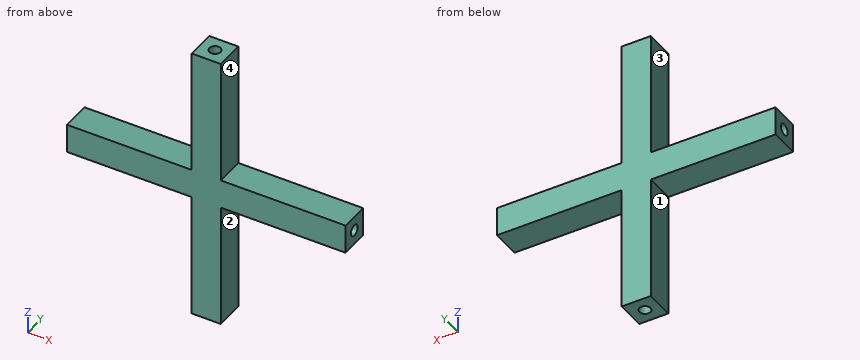
from build123d import *

# Parameters (mm, degrees)
BOSS_EXTRUDE1_DEPTH = 1.75
CUT_EXTRUDE4_START  = -1.75
SKETCH2_R           = 0.675
CUT_EXTRUDE4_DEPTH  = 16
CUT_EXTRUDE5_START  = 1.75
SKETCH2_2_R         = 0.675
CUT_EXTRUDE5_DEPTH  = 16
CUT_EXTRUDE6_START  = 1.75
SKETCH3_R           = 0.675
CUT_EXTRUDE6_DEPTH  = 16
CUT_EXTRUDE7_START  = -1.75
SKETCH3_2_R         = 0.675
CUT_EXTRUDE7_DEPTH  = 16


with BuildPart() as part:
    # Sketch1 → Boss-Extrude1 (new body, symmetric)
    with BuildSketch(Plane(origin=(0, 0, 0), x_dir=(1, 0, 0), z_dir=(0, 1, 0))):
        Polygon((1.75, -1.75), (1.75, -16.75), (-1.75, -16.75), (-1.75, -1.75), (-16.75, -1.75), (-16.75, 1.75), (-1.75, 1.75), (-1.75, 16.75), (1.75, 16.75), (1.75, 1.75), (16.75, 1.75), (16.75, -1.75), align=None)
    extrude(amount=BOSS_EXTRUDE1_DEPTH, both=True)

    # Sketch2 → Cut-Extrude4 (cut, through all)
    with BuildSketch(Plane.XY.offset(CUT_EXTRUDE4_START)):
        Circle(SKETCH2_R)
    extrude(amount=-CUT_EXTRUDE4_DEPTH, mode=Mode.SUBTRACT)

    # Sketch2<2> → Cut-Extrude5 (cut, through all)
    with BuildSketch(Plane.XY.offset(CUT_EXTRUDE5_START)):
        Circle(SKETCH2_2_R)
    extrude(amount=CUT_EXTRUDE5_DEPTH, mode=Mode.SUBTRACT)

    # Sketch3 → Cut-Extrude6 (cut, through all)
    with BuildSketch(Plane.ZY.offset(CUT_EXTRUDE6_START)):
        Circle(SKETCH3_R)
    extrude(amount=CUT_EXTRUDE6_DEPTH, mode=Mode.SUBTRACT)

    # Sketch3<2> → Cut-Extrude7 (cut, through all)
    with BuildSketch(Plane.ZY.offset(CUT_EXTRUDE7_START)):
        Circle(SKETCH3_2_R)
    extrude(amount=-CUT_EXTRUDE7_DEPTH, mode=Mode.SUBTRACT)


solid = part.part
Design review of the part built by this model. Coordinates are the model's own, in mm. Face numbers are marked on the shaded views. A direction names the side the tool comes from. Give positions to 0.01 mm unless a question says otherwise; leave off trailing zeros. Loops run counter-clockwise (first coordinate to the right, second up) from the corner with the lowest first, then second, coordinate; pieces in that order, holes last. Notation, with made-up numbers: M -38,-10 L -18,-10 A23 ccw -18,10 Z; hole C -16.75,33 d11. An arc over 180 degrees is marked long. Answer as a JSON object with one key per item and string values.
Item 1: We need section C-C (x = 0). State the section outline as (y, z) points (3 decimals).
Output values:
{"outline": "M -1.75,-16.75 L -0.675,-16.75 L -0.675,-1.75 L 0.675,-1.75 L 0.675,-16.75 L 1.75,-16.75 L 1.75,16.75 L 0.675,16.75 L 0.675,1.75 L -0.675,1.75 L -0.675,16.75 L -1.75,16.75 Z"}
Item 2: For P1, Ø0.8, axis at x = 0, y = 0, coming from the +Z side; P2, Ø1.1, axis at y = 0, z = 0, coming from the +X side; P3, Ø5, axis at x = -3, z = -7.5, coming from the -Y side; P4, Ø1.5, axis at y = 0.5, z = 9.5, coming from the -X side, all flat-tipped, find the tip position at first contact; note any pin that passes through.
Output values:
{"P1": "stops at z = 1.75", "P2": "stops at x = 1.75", "P3": "stops at y = -1.75", "P4": "stops at x = -1.75"}
Item 3: We need section D-D (z = 0). State the section outline as (x, y) points (3 decimals), and give its area (4 significant figures).
Output values:
{"outline": "M -16.75,-1.75 L 16.75,-1.75 L 16.75,-0.675 L 1.75,-0.675 L 1.75,0.675 L 16.75,0.675 L 16.75,1.75 L -16.75,1.75 L -16.75,0.675 L -1.75,0.675 L -1.75,-0.675 L -16.75,-0.675 Z", "area": "76.75 mm2"}
Item 4: Machinability: for the marked faces 1, 2, 3 and 4, which of the approach directions +Z, -Z, +X, -X, +Y, -Y give a long, thin tool a straight path to every point of the face, cutting with its end or side? Answer none if there is none.
Output values:
{"face 1": "-Z, -X, +Y, -Y", "face 2": "-Z, +X, +Y, -Y", "face 3": "+Z, -X, +Y, -Y", "face 4": "+Z, +X, +Y, -Y"}
Item 5: Wall thickness on line 1 along X through (y, z) = (0, 6.75) (3 decimals): over which ranges is the line inside the solid? List them lowest first.
Output values:
{"line 1": "x = -1.75 to -0.675, 0.675 to 1.75"}
Item 6: We need section A-A (x = -4). State the section outline as (y, z) points (3 decimals), and give its area (3 significant figures).
Output values:
{"outline": "M -1.75,-1.75 L 1.75,-1.75 L 1.75,1.75 L -1.75,1.75 Z; hole C 0,0 d1.35", "area": "10.8 mm2"}
